Geometry: final body of the model. Coordinates: model frame, mm. A direction names the side the tool comes from. Give positions to 0.01 mm unless a question says otherwise; leave off trailing zeros. Write each loop counter-clockwise with the first axis right and the second up, starting at its lowest first coordinate (ties: lowest second). Pieces come first, ordered by that corner, then holes. Notation, with made-up numbers: (18.25, 27.25) - (51.25, 27.25) arc R21 ccw to (51.25, 61.25) - close; hole circle Ø8 at (80.5, -23.5). An arc over 180 degrees is marked (long way). Return JSON: item names as keys, results as strings.
Autodesk Inventor part; units mm, degrees
ref_plane "YZ Plane" through (0, 0, 0) normal (1, 0, 0) x (0, 1, 0)
ref_plane "XZ Plane" through (0, 0, 0) normal (0, 1, 0) x (-1, 0, 0)
ref_plane "XY Plane" through (0, 0, 0) normal (0, 0, 1) x (1, 0, 0)
sketch "Sketch1" plane through (0, 0, 0) normal (0, 1, 0) x (-1, 0, 0)
  circle A0 centre (0, 0) radius 12.5
  dimension "d0" = 25
extrude "Extrusion1" add sketch "Sketch1" along normal blind 39.4
hole "ReliefTop" at (0, 39.4, 0) direction (0, -1, 0) diameter 13.97 depth 0.254 countersink diameter 14.478 countersink angle 90
hole "ReliefBottom" at (0, 0, 0) direction (0, 1, 0) diameter 13.97 depth 0.254 countersink diameter 14.478 countersink angle 90
hole "MountBottomM6" at (0, 0.254, 0) direction (0, 1, 0) diameter 4.917 depth 7.366 tip angle 118 countersink diameter 5.508 countersink angle 90
hole "MountTopM4" at (0, 39.146, 0) direction (0, -1, 0) diameter 3.242 depth 14.478 tip angle 118 countersink diameter 3.808 countersink angle 90
sketch "Sketch2" plane through (0, 0, 0) normal (0, 0, 1) x (1, 0, 0)
  circle A0 centre (0, 20) radius 3
  line L0 (-12.5, 0) -> (12.5, 0)
  line L1 (0, -4.6) -> (0, 27.6)
  point P0 (0, 0)
  dimension "d49" = 6
  dimension "d50" = 20
extrude "Extrusion2" cut sketch "Sketch2" along normal through all both and the other way through all
chamfer "Chamfer1" distance 0.313 angle 45 2 edges at (-3, 19.9998, 12.1347) (-3, 19.9998, -12.1347)
equation "\"d1\" = height"
equation "\"d5\" = reliefMinor"
equation "\"d7\" = reliefMajor"
equation "\"d10\" = reliefDepth"
equation "\"d14\" = reliefMinor"
equation "\"d16\" = reliefMajor"
equation "\"d19\" = reliefDepth"
equation "\"d25\" = chamferM6"
equation "\"d28\" = depthM6"
equation "\"d40\" = chamferM4"
equation "\"d43\" = depthM4"
equation "\"reliefDepth\" = 0.254"
equation "\"reliefMinor\" = 13.97"
equation "\"reliefMajor\" = 14.478"
equation "\"chamferM6\" = 5.508"
equation "\"chamferM4\" = 3.808"
equation "\"depthM6\" = 7.366"
equation "\"depthM4\" = 14.478"
equation "\"height\" = 39.4"
properties part number "PLS-P642H0394A00_M" material "Stainless Steel"
Q1. Section query C-C, the plane x = 10.75. Return the cut outline in (y, z), plus the area to 3 significant figures.
Answer key:
{"outline": "(0, -6.38) - (39.4, -6.38) - (39.4, 6.38) - (0, 6.38) - close", "area": "503 mm^2"}
Q2. Mould query, pull axis X, two halves, no side actions, for faces 1 (the cylindrical face through (-11.923, 19.424, -3.755)), 2 (the flat face through (-5.4, 39.4, -5.4)), 3 (the cylindrical face through (1.438, 31.666, 0.748)). Classes: pulls with the +X half, pulls with the -X half, needs draft (parallel to the pull), parting line crosses it, or undercut.
Answer key:
{"face 1": "parting line crosses it", "face 2": "needs draft", "face 3": "undercut"}
Q3. Section query D-D, the plane x = -9. Return the cut outline in (y, z), plus the area to 3 significant figures.
Answer key:
{"outline": "(0, -8.67) - (39.4, -8.67) - (39.4, 8.67) - (0, 8.67) - close", "area": "684 mm^2"}
Q4. Pin query (flat end, axial travel): P1, Ø5, axis at x = 3, z = 3.5, coming from the -Y side; P2, Ø6, axis at x = -3.5, y = 6, coming from the -Z side; P3, Ø4, axis at x = 0, z = 0, coming from the -Y side; P4, Ø5.5, axis at x = 0, y = 20, coming from the -Z side. Return the tip coordinate at first contact, or that it passes through.
Answer key:
{"P1": "stops at y = 0.13", "P2": "stops at z = -12.49", "P3": "stops at y = 7.9", "P4": "passes through"}
Q5. Set-up query: faces 4 (the cylindrical face through (-0.65, 17.07, 0.17)), 5 (the flat face through (1.5, 39.146, 1.5)), 6 (the flat face through (0, 0.254, -3)). Return all of +Z, -Z, +X, -X, +Y, -Y with unobstructed straight access to the full face (end or side cutting, diameter ignored); none if empty.
Answer key:
{"face 4": "+Z, -Z", "face 5": "+Y", "face 6": "-Y"}
Q6. Section query B-B, the plane y = 15. Return the cut outline in (x, z), plus the area to 3 significant figures.
Answer key:
{"outline": "circle Ø25 at (0, 0)", "area": "491 mm^2"}
Q7. Material intervals for probe 1 along Z at (x, y) = (0, 6); probe 2 along X at (y, z) = (14, 0.5); probe 3 along Y at (x, z) = (0, 2), sorted ascending. Write a range as [from, to].
Answer key:
{"probe 1": "z = [-12.5, -2.46], [2.46, 12.5]", "probe 2": "x = [-12.49, 12.49]", "probe 3": "y = [7.9, 17], [23, 39.15]"}
Q8. Section query A-A, the plane y = 36. Return the cut outline in (x, z).
Answer key:
{"outline": "circle Ø25 at (0, 0); hole circle Ø3.24 at (0, 0)"}
